The listing builds one solid part. Answer for the finished solid, in the listing's coordinates (mm). Face numbers are marked on the shaded views. A direction names the side the tool comes from. Round coordinates to 2 decimals unless told otherwise and drop trailing zeros. Write each loop counter-clockwise with the first axis right and the second up, starting at its lowest first coordinate (ties: lowest second). Pieces come first, ordered by that corner, then holes. Notation, with made-up numbers: M 35.5,58.5 L 88.5,58.5 A18 cw 88.5,72.5 Z; hole C -5.5,-22 d1. An arc over 180 degrees is marked long. Put each result on its own line as item: value. Start each with the question number.
```python
from build123d import *

# Parameters (mm, degrees)
SKETCH1_W               = 36.068
SKETCH1_H               = 38.1
BOSS_EXTRUDE1_DEPTH     = 63.5
SKETCH3_W               = 36.068
SKETCH3_H               = 10.16
CUT_EXTRUDE1_DEPTH      = 38.1
SKETCH4_W               = 36.068
SKETCH4_H               = 17.145
CUT_EXTRUDE2_DEPTH      = 19.05
SKETCH5_W               = 17.399
SKETCH5_H               = 10.16
CUT_EXTRUDE3_DEPTH      = 47.257298408
CUT_EXTRUDE4_DEPTH      = 71.283227416
CUT_EXTRUDE4_DEPTH_BACK = 71.283227416
SKETCH6_R               = 1.125
BOSS_EXTRUDE2_REACH     = 70.705
SKETCH7_W               = 8.509
SKETCH7_H               = 38.1
SKETCH8_W               = 10.16
SKETCH8_H               = 6.35
BOSS_EXTRUDE3_DEPTH     = 8.89


with BuildPart() as part:
    # Sketch1 → Boss-Extrude1 (new body)
    with BuildSketch(Plane(origin=(0, 0, 0), x_dir=(1, 0, 0), z_dir=(0, 1, 0))):
        Rectangle(SKETCH1_W, SKETCH1_H)
    extrude(amount=BOSS_EXTRUDE1_DEPTH)

    # Sketch3 → Cut-Extrude1 (cut)
    with BuildSketch(Plane(origin=(0, 63.5, 0), x_dir=(1, 0, 0), z_dir=(0, 1, 0))):
        Rectangle(SKETCH3_W, SKETCH3_H)
    extrude(amount=-CUT_EXTRUDE1_DEPTH, mode=Mode.SUBTRACT)

    # Sketch4 → Cut-Extrude2 (cut)
    with BuildSketch(Plane.XZ):
        Rectangle(SKETCH4_W, SKETCH4_H)
    extrude(amount=-CUT_EXTRUDE2_DEPTH, mode=Mode.SUBTRACT)

    # Sketch5 → Cut-Extrude3 (cut, through all)
    with BuildSketch(Plane(origin=(0, 25.4, 0), x_dir=(1, 0, 0), z_dir=(0, 1, 0))):
        with Locations((-9.3345, 0)):
            Rectangle(SKETCH5_W, SKETCH5_H)
        with Locations((9.3345, 0)):
            Rectangle(SKETCH5_W, SKETCH5_H)
    extrude(amount=-CUT_EXTRUDE3_DEPTH, mode=Mode.SUBTRACT)

    # Sketch6 → Cut-Extrude4 (cut, two sides: drawn at the far end of the back side and taken through both)
    with BuildSketch(Plane.XY.offset(-5.08).offset(-CUT_EXTRUDE4_DEPTH_BACK)):
        with Locations((0, 29.845)):
            Circle(SKETCH6_R)
    extrude(amount=CUT_EXTRUDE4_DEPTH + CUT_EXTRUDE4_DEPTH_BACK, mode=Mode.SUBTRACT)

    # Boss-Extrude2: up to this face of the body (flat: up to its plane)
    boss_extrude2_end = Plane(part.part.faces().sort_by_distance((0, 0, 13.81125))[0])
    # Sketch7 → Boss-Extrude2 (add, up to the picked face)
    with BuildSketch(Plane(origin=(0, 63.5, 0), x_dir=(1, 0, 0), z_dir=(0, 1, 0)), mode=Mode.PRIVATE) as boss_extrude2_sk1:
        with Locations((13.7795, 0)):
            Rectangle(SKETCH7_W, SKETCH7_H)
    boss_extrude2_tool1 = split(extrude(boss_extrude2_sk1.sketch, amount=-BOSS_EXTRUDE2_REACH, mode=Mode.PRIVATE), bisect_by=boss_extrude2_end, keep=Keep.BOTH, mode=Mode.PRIVATE)
    add(boss_extrude2_tool1.solids().sort_by(Axis((13.7795, 63.5, 0), (0, -1, 0)))[0])

    # Sketch8 → Boss-Extrude3 (add)
    with BuildSketch(Plane(origin=(0.635, 0, 0), x_dir=(0, 0, -1), z_dir=(1, 0, 0))):
        with Locations((0, 22.225)):
            Rectangle(SKETCH8_W, SKETCH8_H)
    extrude(amount=BOSS_EXTRUDE3_DEPTH)


solid = part.part
```
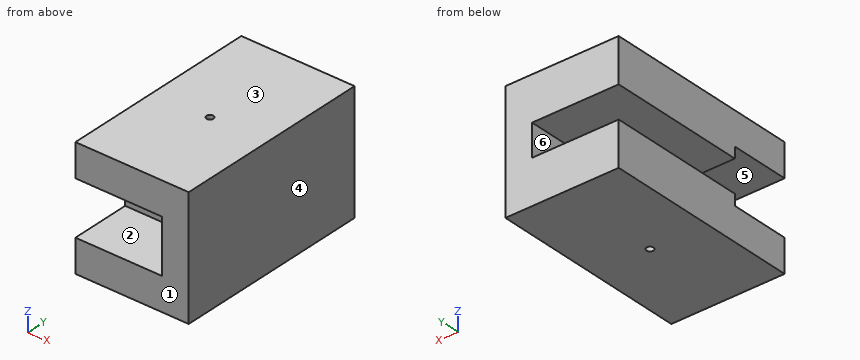
Item 1: Determine the mould class of the marked faces 1, 2 and 3 for opening direction Z: released by +Z, released by -Z, zero draft, split by the parting line, or undercut.
Item 2: Section A-A (x = -7.5) is taken. Give the vertices of the cut face in (y, z), and give its area (3 significant figures).
Item 3: Consider line 1 along Y through (x, z) = (0, -11.5); line 2 along Z through (x, y) = (-12, 48); line 3 along Z through (x, y) = (-7, 16.5). Determine where each line is inside the solid, lowest interval first. Write a range as [from, to].
Item 4: Flat-ended cylindrical pins translate along their axes: pin 1 (5 mm diameter, centred on y = 35.5, z = -0.5, fed in from -X) (3 decimals); pin 2 (3 mm diameter, centred on y = 22.5, z = -2, fed in from -X) (3 decimals). Find the tip coordinate at first contact, or state that the pin passes through.
Item 5: Section B-B (y = 34) is taken. Give the vertices of the cut face in (x, z) (3 decimals).
Item 6: Which of the six approach directions +Z, -Z, +X, -X, +Y, -Y give full straight-line access (tool end or side, diameter ignored) to the marked faces 4, 5 and 6?
Output values:
1. face 1: zero draft
1. face 2: undercut
1. face 3: released by +Z
2. outline: M 0,-19.05 L 63.5,-19.05 L 63.5,-5.08 L 19.05,-5.08 L 19.05,-8.57 L 0,-8.57 Z; M 0,8.57 L 19.05,8.57 L 19.05,5.08 L 63.5,5.08 L 63.5,19.05 L 0,19.05 Z
2. area: 1,640 mm^2
3. line 1: y = [0, 28.72], [30.97, 63.5]
3. line 2: z = [-19.05, -5.08], [5.08, 19.05]
3. line 3: z = [-19.05, -8.57], [8.57, 19.05]
4. pin 1: stops at x = 9.525
4. pin 2: stops at x = -0.635
5. outline: M -18.034,-19.05 L 18.034,-19.05 L 18.034,19.05 L -18.034,19.05 L -18.034,5.08 L 9.525,5.08 L 9.525,-5.08 L -18.034,-5.08 Z
6. face 4: +Z, -Z, +X, +Y, -Y
6. face 5: -X, -Y
6. face 6: -X, +Y
